```python
from build123d import *

# Parameters (mm, degrees)
SKETCH1_W           = 20
SKETCH1_H           = 50
BOSS_EXTRUDE1_DEPTH = 5
SKETCH2_R           = 1.6
CUT_EXTRUDE1_DEPTH  = 28.386127875
SKETCH3_W           = 20
SKETCH3_H           = 10
SKETCH3_H_2         = 7
BOSS_EXTRUDE2_DEPTH = 5
SKETCH4_R           = 1.45
CUT_EXTRUDE2_DEPTH  = 34.541019662
SKETCH5_W           = 6.666666666
SKETCH5_H           = 5
CUT_EXTRUDE3_DEPTH  = 52.961524227
CUT_EXTRUDE4_REACH  = 35.541
SKETCH6_R           = 1.6
FILLET1_R           = 2


with BuildPart() as part:
    # Sketch1 → Boss-Extrude1 (new body)
    with BuildSketch(Plane(origin=(0, 0, 0), x_dir=(1, 0, 0), z_dir=(0, 1, 0))):
        Rectangle(SKETCH1_W, SKETCH1_H)
    extrude(amount=BOSS_EXTRUDE1_DEPTH)

    # Sketch2 → Cut-Extrude1 (cut, through all)
    with BuildSketch(Plane(origin=(0, 5, 0), x_dir=(1, 0, 0), z_dir=(0, 1, 0))):
        with Locations(Location((0, 12.5, 0), (0, 0, 270))):
            Circle(SKETCH2_R)
        with Locations(Location((0, -12.5, 0), (0, 0, 270))):
            Circle(SKETCH2_R)
    extrude(amount=-CUT_EXTRUDE1_DEPTH, mode=Mode.SUBTRACT)

    # Sketch3 → Boss-Extrude2 (add)
    with BuildSketch(Plane(origin=(0, 5, 0), x_dir=(1, 0, 0), z_dir=(0, 1, 0))):
        Rectangle(SKETCH3_W, SKETCH3_H)
        with Locations((0, -21.5)):
            Rectangle(SKETCH3_W, SKETCH3_H_2)
        with Locations((0, 21.5)):
            Rectangle(SKETCH3_W, SKETCH3_H_2)
    extrude(amount=BOSS_EXTRUDE2_DEPTH)

    # Sketch4 → Cut-Extrude2 (cut, through all)
    with BuildSketch(Plane.ZY.offset(10)):
        with Locations((-21.5, 7.5)):
            Circle(SKETCH4_R)
        with Locations((0, 7.5)):
            Circle(SKETCH4_R)
        with Locations((21.5, 7.5)):
            Circle(SKETCH4_R)
    extrude(amount=-CUT_EXTRUDE2_DEPTH, mode=Mode.SUBTRACT)

    # Sketch5 → Cut-Extrude3 (cut, through all)
    with BuildSketch(Plane(origin=(0, 0, -25), x_dir=(-1, 0, 0), z_dir=(0, 0, -1))):
        with Locations((0, 7.5)):
            Rectangle(SKETCH5_W, SKETCH5_H)
    extrude(amount=-CUT_EXTRUDE3_DEPTH, mode=Mode.SUBTRACT)

    # Sketch6 → Cut-Extrude4 (cut, up to next)
    with BuildSketch(Plane(origin=(10, 0, 0), x_dir=(0, 0, -1), z_dir=(1, 0, 0)), mode=Mode.PRIVATE) as cut_extrude4_sk1:
        with Locations((21.5, 7.5)):
            Circle(SKETCH6_R)
    cut_extrude4_tool1 = extrude(cut_extrude4_sk1.sketch, amount=-CUT_EXTRUDE4_REACH, mode=Mode.PRIVATE) & part.part
    # Sketch6 → Cut-Extrude4 (cut, up to next)
    with BuildSketch(Plane(origin=(10, 0, 0), x_dir=(0, 0, -1), z_dir=(1, 0, 0)), mode=Mode.PRIVATE) as cut_extrude4_sk2:
        with Locations((0, 7.5)):
            Circle(SKETCH6_R)
    cut_extrude4_tool2 = extrude(cut_extrude4_sk2.sketch, amount=-CUT_EXTRUDE4_REACH, mode=Mode.PRIVATE) & part.part
    # Sketch6 → Cut-Extrude4 (cut, up to next)
    with BuildSketch(Plane(origin=(10, 0, 0), x_dir=(0, 0, -1), z_dir=(1, 0, 0)), mode=Mode.PRIVATE) as cut_extrude4_sk3:
        with Locations((-21.5, 7.5)):
            Circle(SKETCH6_R)
    cut_extrude4_tool3 = extrude(cut_extrude4_sk3.sketch, amount=-CUT_EXTRUDE4_REACH, mode=Mode.PRIVATE) & part.part
    add(cut_extrude4_tool1.solids().sort_by_distance((10, 7.5, -21.5))[0], mode=Mode.SUBTRACT)
    add(cut_extrude4_tool2.solids().sort_by_distance((10, 7.5, 0))[0], mode=Mode.SUBTRACT)
    add(cut_extrude4_tool3.solids().sort_by_distance((10, 7.5, 21.5))[0], mode=Mode.SUBTRACT)

    # Fillet1
    fillet1_edges = [part.edges().sort_by_distance(p)[0] for p in [
        (6.666666667, 10, -25),
        (-6.666666667, 10, -18),
        (6.666666667, 10, 18),
        (-6.666666667, 10, 25),
        (6.666666667, 10, -5),
        (-6.666666667, 10, 5),
        (-6.666666667, 10, -25),
        (6.666666667, 10, -18),
        (-6.666666667, 10, 18),
        (6.666666667, 10, 25),
        (-6.666666667, 10, -5),
        (6.666666667, 10, 5),
    ]]
    fillet(fillet1_edges, radius=FILLET1_R)


solid = part.part
```
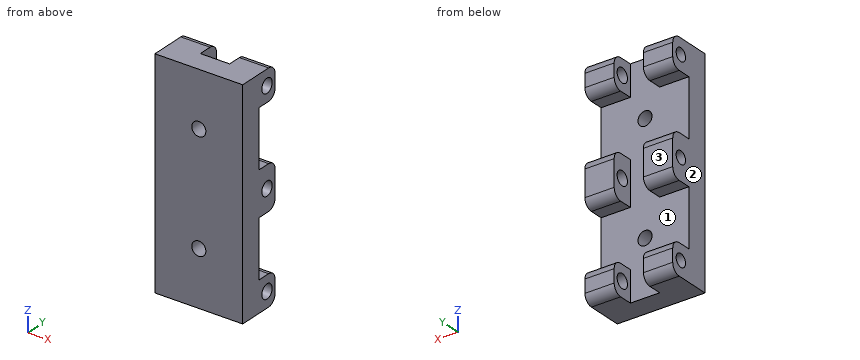
CAD build for the part. Positions are in the model's coordinates, mm. Face numbers are marked on the shaded views. Coordinates: 2 decimals unless noted, no trailing zeros. Order: outer loops, then holes, each group sorted by start corner. A loop starts at its lowest first (then second) coordinate and runs counter-clockwise, first axis right, second up. Notation, with made-up numbers: (-39, -23) - (-18, -23) arc R19 cw to (-18, 12) - close; hole circle Ø6 at (63, 78.5). An arc over 180 degrees is marked (long way). Use a Markdown table: item, result. Add a question column.
(1) Saw through at C-C (z = 0). Give the cut face in (x, y).
(2) Flat gauge pins, fed straight in: pin 1 (3.5 mm diameter, centred on y = 7.5, z = -21.5, fed in from +X); pin 2 (10 mm diameter, centred on x = 2.5, z = 10, fed in from +Y). Where does each tip first touch, or does it go through?
(3) Drill centre lines: line 1 along Z through (x, y) = (-7.5, 6); line 2 along Y through (x, z) = (-7, 0); line 3 along X through (y, z) = (5.25, 19). Where is each one in solid material? Low to high. Write a range as [from, to].
(4) Saw through at A-A (z = -12.5). Give the cut face in (x, y).
(5) Saw through at B-B (x = 6.5). Give the cut face in (y, z).
(6) Saw through at D-D (y = 3.75). Give the cut face in (x, z), then the cut area to 3 significant figures.
(7) Pull direction X, two halves, no side cores. Call the marked faces 1, 2 and 3: +X half, -X half, draft (parallel to the pull), parting line (faces both ways), or undercut.
Solved:
| question | item | result |
|---|---|---|
| 1 | outline | (-10, 0) - (10, 0) - (10, 5.9) - (3.33, 5.9) - (3.33, 5) - (-3.33, 5) - (-3.33, 6.05) - (-10, 6.05) - close; (-10, 8.95) - (-3.33, 8.95) - (-3.33, 10) - (-10, 10) - close; (3.33, 9.1) - (10, 9.1) - (10, 10) - (3.33, 10) - close |
| 2 | pin 1 | stops at x = 10 |
| 2 | pin 2 | stops at y = 5 |
| 3 | line 1 | z = [-25, -18], [-5, 5], [18, 25] |
| 3 | line 2 | y = [0, 6.05], [8.95, 10] |
| 3 | line 3 | x = [-10, -3.33], [3.33, 10] |
| 4 | outline | (-10, 0) - (-1.6, 0) - (-1.6, 5) - (-10, 5) - close; (1.6, 0) - (10, 0) - (10, 5) - (1.6, 5) - close |
| 5 | outline | (0, -25) - (8, -25) arc R2 ccw to (10, -23) - (10, -20) arc R2 ccw to (8, -18) - (5, -18) - (5, -5) - (8, -5) arc R2 ccw to (10, -3) - (10, 3) arc R2 ccw to (8, 5) - (5, 5) - (5, 18) - (8, 18) arc R2 ccw to (10, 20) - (10, 23) arc R2 ccw to (8, 25) - (0, 25) - close; hole circle Ø3.2 at (7.5, -21.5); hole circle Ø3.2 at (7.5, 0); hole circle Ø3.2 at (7.5, 21.5) |
| 6 | outline | (-10, -25) - (10, -25) - (10, 25) - (-10, 25) - close; hole circle Ø3.2 at (0, -12.5); hole circle Ø3.2 at (0, 12.5) |
| 6 | area | 984 mm² |
| 7 | face 1 | undercut |
| 7 | face 2 | -X half |
| 7 | face 3 | draft |
